Geometry check sheet. Reference: the model listing, model coordinates, mm. Coordinates: 2 decimals unless noted, no trailing zeros. Write each loop counter-clockwise with the first axis right and the second up, starting at its lowest first coordinate (ties: lowest second). Pieces come first, ordered by that corner, then holes.
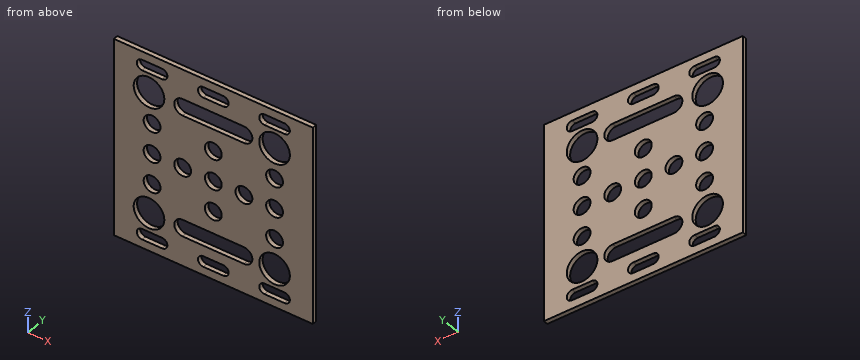
from build123d import *

# Parameters (mm, degrees)
SKETCH1_W           = 65
SKETCH1_H           = 65
SKETCH1_R           = 2.75
SKETCH1_R_2         = 5
BOSS_EXTRUDE1_DEPTH = 1.5


with BuildPart() as part:
    # Sketch1 → Boss-Extrude1 (new body)
    with BuildSketch(Plane(origin=(0, 0, 0), x_dir=(1, 0, 0), z_dir=(0, 1, 0))):
        with Locations((32.5, 32.5)):
            Rectangle(SKETCH1_W, SKETCH1_H)
        with Locations((32.5, 32.5)):
            Circle(SKETCH1_R, mode=Mode.SUBTRACT)
        with Locations((22.5, 32.5)):
            Circle(SKETCH1_R, mode=Mode.SUBTRACT)
        with Locations((12.5, 32.5)):
            Circle(SKETCH1_R, mode=Mode.SUBTRACT)
        with Locations((32.5, 42.5)):
            Circle(SKETCH1_R, mode=Mode.SUBTRACT)
        with Locations((12.5, 42.5)):
            Circle(SKETCH1_R, mode=Mode.SUBTRACT)
        with Locations((11.5, 52.5)):
            Circle(SKETCH1_R_2, mode=Mode.SUBTRACT)
        with Locations((42.5, 32.5)):
            Circle(SKETCH1_R, mode=Mode.SUBTRACT)
        with Locations((52.5, 32.5)):
            Circle(SKETCH1_R, mode=Mode.SUBTRACT)
        with Locations((52.5, 42.5)):
            Circle(SKETCH1_R, mode=Mode.SUBTRACT)
        with Locations((52.5, 22.5)):
            Circle(SKETCH1_R, mode=Mode.SUBTRACT)
        with Locations((32.5, 22.5)):
            Circle(SKETCH1_R, mode=Mode.SUBTRACT)
        with Locations((12.5, 22.5)):
            Circle(SKETCH1_R, mode=Mode.SUBTRACT)
        with Locations((11.5, 12.5)):
            Circle(SKETCH1_R_2, mode=Mode.SUBTRACT)
        with Locations((52.5, 52.5)):
            Circle(SKETCH1_R_2, mode=Mode.SUBTRACT)
        with Locations((52.5, 12.5)):
            Circle(SKETCH1_R_2, mode=Mode.SUBTRACT)
        with BuildLine():
            Line((22.5, 55.25), (42.5, 55.25))
            ThreePointArc((42.5, 55.25), (45.25, 52.5), (42.5, 49.75))
            Line((42.5, 49.75), (22.5, 49.75))
            ThreePointArc((22.5, 49.75), (19.75, 52.5), (22.5, 55.25))
        make_face(mode=Mode.SUBTRACT)
        with BuildLine():
            Line((29.25, 62.25), (35.75, 62.25))
            ThreePointArc((35.75, 62.25), (37.5, 60.5), (35.75, 58.75))
            Line((35.75, 58.75), (29.25, 58.75))
            ThreePointArc((29.25, 58.75), (27.5, 60.5), (29.25, 62.25))
        make_face(mode=Mode.SUBTRACT)
        with BuildLine():
            Line((9.25, 62.25), (15.75, 62.25))
            ThreePointArc((15.75, 62.25), (17.5, 60.5), (15.75, 58.75))
            Line((15.75, 58.75), (9.25, 58.75))
            ThreePointArc((9.25, 58.75), (7.5, 60.5), (9.25, 62.25))
        make_face(mode=Mode.SUBTRACT)
        with BuildLine():
            Line((55.75, 62.25), (49.25, 62.25))
            ThreePointArc((49.25, 62.25), (47.5, 60.5), (49.25, 58.75))
            Line((49.25, 58.75), (55.75, 58.75))
            ThreePointArc((55.75, 58.75), (57.5, 60.5), (55.75, 62.25))
        make_face(mode=Mode.SUBTRACT)
        with BuildLine():
            Line((22.5, 9.75), (42.5, 9.75))
            ThreePointArc((42.5, 9.75), (45.25, 12.5), (42.5, 15.25))
            Line((42.5, 15.25), (22.5, 15.25))
            ThreePointArc((22.5, 15.25), (19.75, 12.5), (22.5, 9.75))
        make_face(mode=Mode.SUBTRACT)
        with BuildLine():
            Line((55.75, 2.75), (49.25, 2.75))
            ThreePointArc((49.25, 2.75), (47.5, 4.5), (49.25, 6.25))
            Line((49.25, 6.25), (55.75, 6.25))
            ThreePointArc((55.75, 6.25), (57.5, 4.5), (55.75, 2.75))
        make_face(mode=Mode.SUBTRACT)
        with BuildLine():
            Line((9.25, 2.75), (15.75, 2.75))
            ThreePointArc((15.75, 2.75), (17.5, 4.5), (15.75, 6.25))
            Line((15.75, 6.25), (9.25, 6.25))
            ThreePointArc((9.25, 6.25), (7.5, 4.5), (9.25, 2.75))
        make_face(mode=Mode.SUBTRACT)
        with BuildLine():
            Line((29.25, 2.75), (35.75, 2.75))
            ThreePointArc((35.75, 2.75), (37.5, 4.5), (35.75, 6.25))
            Line((35.75, 6.25), (29.25, 6.25))
            ThreePointArc((29.25, 6.25), (27.5, 4.5), (29.25, 2.75))
        make_face(mode=Mode.SUBTRACT)
    extrude(amount=BOSS_EXTRUDE1_DEPTH)


solid = part.part
1. Sectioned sample at B-B, the plane x = 32.5. Give the number of separate pieces and of enclosed holes in the cut face, and give its area (4 significant figures).
Computed values:
separate pieces: 8
enclosed holes: 0
area: 45.75 mm2
2. Thickness scan on line 1 along X through (y, z) = (0.3, -42.5); line 2 along Z through (x, y) = (29, 1.15); line 3 along Z through (x, y) = (45, 0.2). Record the ranges inside material, lowest first.
Computed values:
line 1: x = 0 to 9.75, 15.25 to 29.75, 35.25 to 49.75, 55.25 to 65
line 2: z = -65 to -62.23, -58.77 to -55.25, -49.75 to -15.25, -9.75 to -6.23, -2.77 to 0
line 3: z = -65 to -53.65, -51.35 to -33.65, -31.35 to -13.65, -11.35 to 0
3. Sectioned sample at C-C, the plane z = -12.5. Record the boundary of the cut face in (x, y).
Computed values:
outline: (0, 0) - (6.5, 0) - (6.5, 1.5) - (0, 1.5) - close; (16.5, 0) - (19.75, 0) - (19.75, 1.5) - (16.5, 1.5) - close; (45.25, 0) - (47.5, 0) - (47.5, 1.5) - (45.25, 1.5) - close; (57.5, 0) - (65, 0) - (65, 1.5) - (57.5, 1.5) - close
4. Sectioned sample at A-A, the plane z = -32.5. Record the boundary of the cut face in (x, y).
Computed values:
outline: (0, 0) - (9.75, 0) - (9.75, 1.5) - (0, 1.5) - close; (15.25, 0) - (19.75, 0) - (19.75, 1.5) - (15.25, 1.5) - close; (25.25, 0) - (29.75, 0) - (29.75, 1.5) - (25.25, 1.5) - close; (35.25, 0) - (39.75, 0) - (39.75, 1.5) - (35.25, 1.5) - close; (45.25, 0) - (49.75, 0) - (49.75, 1.5) - (45.25, 1.5) - close; (55.25, 0) - (65, 0) - (65, 1.5) - (55.25, 1.5) - close
